Work out the finished part from the listing and answer in its coordinate system (mm). Face numbers are marked on the shaded views. A direction names the side the tool comes from. Round coordinates to 2 decimals unless told otherwise and drop trailing zeros. Loops run counter-clockwise (first coordinate to the right, second up) from the corner with the lowest first, then second, coordinate; pieces in that order, holes last. Notation, with made-up numbers: M 78.5,17.25 L 130.5,17.25 A8 ccw 130.5,24.25 Z; hole C 56,29.5 d10. An arc over 180 degrees is marked long. One line per item, written item: value.
Autodesk Inventor part; units mm, degrees
ref_plane "YZ Plane" through (0, 0, 0) normal (1, 0, 0) x (0, 1, 0)
ref_plane "XZ Plane" through (0, 0, 0) normal (0, 1, 0) x (-1, 0, 0)
ref_plane "XY Plane" through (0, 0, 0) normal (0, 0, 1) x (1, 0, 0)
sketch "スケッチ1" plane through (0, 0, 0) normal (1, 0, 0) x (0, 1, 0)
  line L0 (-20, 24) -> (63.1384, 24)
  line L1 (63.1384, 24) -> (63.1384, -24)
  line L2 (25, -24) -> (-20, -24)
  line L3 (-20, -24) -> (-20, 24)
  line L4 (-20, 24) -> (63.1384, -24)
  line L5 (-20, -24) -> (25, -24)
  line L6 (25, -24) -> (25, -1.9808)
  line L7 (25, 24) -> (-20, 24)
  line L8 (-20, 24) -> (-20, -24)
  point P0 (0, 0)
  dimension "d6" = 24
  dimension "d7" = 48
  dimension "d96" = 45
  dimension "d98" = 83.1384
extrude "押し出し1" add sketch "スケッチ1" along normal blind 28 contours L4 L6 L2 L3
sketch "スケッチ2" plane through (28, 0, 0) normal (1, 0, 0) x (0, 0, -1)
  line L0 (-6.6795, -10) -> (14, -10)
  line L1 (14, -10) -> (14, 25.8179)
  line L2 (14, 25.8179) -> (-6.6795, 25.8179)
  line L3 (-6.6795, 25.8179) -> (-6.6795, 13)
  line L4 (-24, -20) -> (24, -20)
  line L5 (24, -20) -> (24, 25)
  line L6 (-6.6795, -10) -> (14, 25.8179)
  line L7 (14, -10) -> (-6.679, -10)
  line L8 (-6.679, -10) -> (-6.679, 13)
  line L9 (6.5996, 13) -> (14, 13)
  line L10 (14, 13) -> (14, -10)
  point P0 (0, 0)
  point P1 (24, 63.1384)
  dimension "d10" = 20.6795
  dimension "d11" = 35.8179
  dimension "d12" = 10
  dimension "d13" = 10
  dimension "d19" = 20.679
  dimension "d75" = 23
extrude "押し出し2" cut sketch "スケッチ2" against normal blind 40 contours L6 L9 L1 L0
sketch "スケッチ3" plane through (28, -10, 6.6795) normal (0, 1, 0) x (1, 0, 0)
  line L0 (0, 20.6795) -> (0, 0)
  line L1 (0, 20.6795) -> (-28, 20.6795)
  line L2 (-19.1, 5.5795) -> (-8.9, 5.5795)
  line L3 (-8.9, 5.5795) -> (-8.9, 19.7795)
  line L4 (-8.9, 19.7795) -> (-19.1, 19.7795)
  line L5 (-19.1, 19.7795) -> (-19.1, 5.5795)
  line L6 (-22.6, 8.4295) -> (-5.4, 8.4295)
  line L7 (-5.4, 8.4295) -> (-5.4, 16.9295)
  line L8 (-5.4, 16.9295) -> (-22.6, 16.9295)
  line L9 (-22.6, 16.9295) -> (-22.6, 8.4295)
  point P0 (-28, 6.6795)
  point P1 (-14, 12.6795)
  dimension "d16" = 14
  dimension "d17" = 8
  dimension "d21" = 10.2
  dimension "d22" = 14.2
  dimension "d23" = 7.1
  dimension "d24" = 5.1
  dimension "d25" = 17.2
  dimension "d26" = 8.5
  dimension "d27" = 4.25
  dimension "d28" = 8.6
extrude "押し出し3" cut sketch "スケッチ3" against normal blind 5
sketch "スケッチ4" plane through (28, -15, 6.6795) normal (0, 1, 0) x (1, 0, 0)
  line L0 (0, 20.6795) -> (-28, 20.6795)
  line L1 (0, 20.6795) -> (0, 0)
  circle A0 centre (-14, 12.6795) radius 2.6
  point P0 (-28, 6.6795)
  dimension "d31" = 8
  dimension "d32" = 14
  dimension "d33" = 5.2
extrude "押し出し4" cut sketch "スケッチ4" against normal blind 5
fillet "フィレット1" radius 1 4 edges at (8.9, -12.5, -10.25) (8.9, -12.5, -1.75) (19.1, -12.5, -10.25) (19.1, -12.5, -1.75)
sketch "スケッチ8" plane through (28, 25.8179, -14) normal (0, -0.5, -0.866) x (-1, 0, 0)
  line L0 (0, -41.359) -> (28, -41.359)
  line L1 (5.4, -35.109) -> (22.6, -35.109)
  line L2 (22.6, -35.109) -> (22.6, -26.609)
  line L3 (22.6, -26.609) -> (5.4, -26.609)
  line L4 (5.4, -26.609) -> (5.4, -35.109)
  line L5 (28, -14.8009) -> (28, -41.359)
  line L6 (8.9, -37.959) -> (19.1, -37.959)
  line L7 (19.1, -37.959) -> (19.1, -23.759)
  line L8 (19.1, -23.759) -> (8.9, -23.759)
  line L9 (8.9, -23.759) -> (8.9, -37.959)
  point P0 (28, -29.359)
  point P1 (14, -30.859)
  dimension "d54" = 10.5
  dimension "d55" = 17.2
  dimension "d56" = 8.5
  dimension "d57" = 14
  dimension "d58" = 8.6
  dimension "d59" = 4.25
  dimension "d60" = 10.2
  dimension "d61" = 14.2
  dimension "d62" = 7.1
  dimension "d63" = 5.1
extrude "押し出し7" cut sketch "スケッチ8" against normal blind 5
sketch "スケッチ9" plane through (28, 28.3179, -9.6699) normal (0, -0.5, -0.866) x (-1, 0, 0)
  line L0 (0, -41.359) -> (28, -41.359)
  line L1 (28, -14.8009) -> (28, -41.359)
  circle A0 centre (14, -30.859) radius 2.6
  point P0 (28, -29.359)
  point P1 (28, 0)
  dimension "d66" = 10.5
  dimension "d67" = 14
  dimension "d68" = 5.2
extrude "押し出し8" cut sketch "スケッチ9" against normal blind 5
fillet "フィレット2" radius 1 4 edges at (19.1, -3.3368, 5.7204) (19.1, 4.0244, 1.4704) (8.9, -3.3368, 5.7204) (8.9, 4.0244, 1.4704)
fillet "フィレット4" radius 1.5 1 edges at (14, -10, 6.6795)
sketch "スケッチ10" plane through (0, 13, -14) normal (0, 0, 1) x (1, 0, 0)
  line L0 (0, -23) -> (0, 0)
  line L1 (28, -23) -> (0, -23)
  line L2 (22.6, -8.25) -> (5.4, -8.25)
  line L3 (5.4, -8.25) -> (5.4, -16.75)
  line L4 (5.4, -16.75) -> (22.6, -16.75)
  line L5 (22.6, -16.75) -> (22.6, -8.25)
  line L6 (19.1, -5.4) -> (8.9, -5.4)
  line L7 (8.9, -5.4) -> (8.9, -19.6)
  line L8 (8.9, -19.6) -> (19.1, -19.6)
  line L9 (19.1, -19.6) -> (19.1, -5.4)
  point P0 (0, -13)
  point P1 (14, -12.5)
  point P2 (0, -22.5)
  dimension "d76" = 14
  dimension "d77" = 10.5
  dimension "d78" = 17.2
  dimension "d79" = 8.5
  dimension "d80" = 8.6
  dimension "d81" = 4.25
  dimension "d82" = 10.2
  dimension "d83" = 14.2
  dimension "d84" = 7.1
  dimension "d85" = 5.1
extrude "押し出し9" cut sketch "スケッチ10" against normal blind 5
sketch "スケッチ11" plane through (0, 13, -19) normal (0, 0, 1) x (1, 0, 0)
  line L0 (28, -23) -> (0, -23)
  line L1 (0, -23) -> (0, 0)
  circle A0 centre (14, -12.5) radius 2.6
  point P0 (0, -13)
  dimension "d88" = 10.5
  dimension "d89" = 14
  dimension "d90" = 5.2
extrude "押し出し10" cut sketch "スケッチ11" against normal blind 5
fillet "フィレット6" radius 0.5 1 edges at (14, -10, -14)
fillet "フィレット8" radius 2 1 edges at (14, 13, -6.5996)
chamfer "面取り1" distance 6 angle 45 1 edges at (14, 25, -24)
fillet "フィレット9" radius 6 1 edges at (14, -20, 24)
fillet "フィレット10" radius 3 1 edges at (14, -20, -24)
fillet "フィレット11" radius 2 1 edges at (14, 25, -1.9808)
chamfer "面取り3" distance 3 angle 45 1 edges at (14, 13, -14)
fillet "フィレット12" radius 1 7 edges at (0, -17, 18.8038) (0, -20, -3.6962) (0, -19.1213, -23.1213) (0, 1, -24) (0, 24.7321, -2.1355) (0, 25, -10.5677) (0, 6.5, 8.7002)
fillet "フィレット13" radius 1 5 edges at (0.2929, 24.7071, -18.2929) (14.5, 25, -18) (0.2929, 19.2929, -23.7071) (14.5, 19, -24) (0, 22, -21)
fillet "フィレット14" radius 1 10 edges at (28, -17, 18.8038) (28, -20, -3.6962) (28, -19.1213, -23.1213) (28, 0.7929, -24) (28, 18.9685, -23.9239) (28, 22, -21) (28, 24.9239, -17.9685) (28, 25, -10.3606) (28, 24.7321, -2.1355) (28, 6.5, 8.7002)
properties part number "triangle_jig"
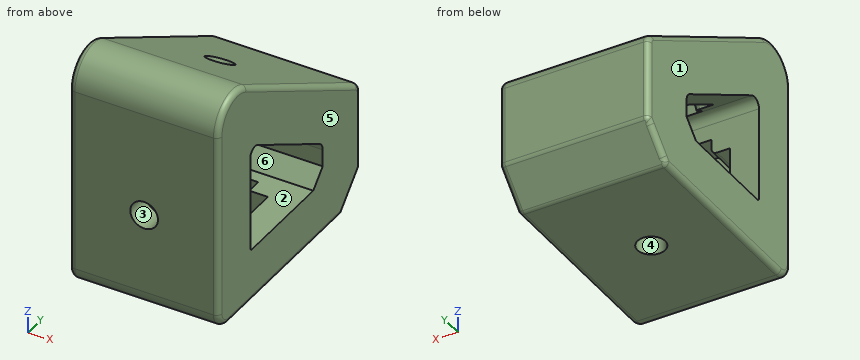
1) Find section D-D (x = 25). Give the vertices of the cut face in (y, z).
Check values:
outline: M -20,-21 A3 ccw -17,-24 L 18.59,-24 A1 ccw 19.29,-23.71 L 24.71,-18.29 A1 ccw 25,-17.59 L 25,-3.14 A2 ccw 24,-1.4 L -11,18.8 A6 ccw -20,13.61 Z; hole M -10,-13.5 A0.5 ccw -9.5,-14 L 10,-14 L 13,-11 L 13,-7.75 A2 ccw 12,-6.02 L -7.75,5.38 A1.5 ccw -10,4.08 Z
2) The mould has two halves that part along X. Classify the marked faces 1, 2 and 3: +X half, -X half, draft (parallel to the pull), parting line (faces both ways), or undercut.
Check values:
face 1: -X half
face 2: draft
face 3: undercut
3) Find section C-C (y = 0.5). Give the number of separate pieces and of enclosed holes in the cut face, then the cut area to 3 significant figures.
Check values:
separate pieces: 3
enclosed holes: 0
area: 382 mm2
4) For the marked faces 4, 5 and 6, determine the directions among +Z, -Z, +X, -X, +Y, -Y from which every point of the face is accessible in a straight line to the end or side of a thin tool.
Check values:
face 4: -Z
face 5: +Z, -Z, +X, +Y, -Y
face 6: +X, -X
5) Find the intervals of material crossed by probe 1 along X at (y, z) = (-16, -6); probe 2 along Y at (x, z) = (14, -23); probe 3 along Z at (x, y) = (22.5, -2.5), in increasing order. Write a range as from..to.
Check values:
probe 1: 0..11.4, 16.6..28
probe 2: -19.24..-2.1, 3.1..20
probe 3: -24..-19, 7.17..13.9
6) Each of these flat-tipped pins is pushed along its axis until it touches: pin 1 (1.2 mm diameter, centred on y = -4, z = 5.5, fed in from -X); pin 2 (1 mm diameter, centred on x = 3, z = -19, fed in from +Y); pin 3 (3 mm diameter, centred on x = 11, z = 15, fed in from +Y); pin 4 (1.5 mm diameter, centred on x = 25, y = 3.5, fed in from +Z). Where does it stop, or does it pass through?
Check values:
pin 1: x = 0
pin 2: y = 24.5
pin 3: y = -1.81
pin 4: z = 10.87
